from build123d import *

# Parameters (mm, degrees)
SKETCH_1_R          = 1.65
SKETCH_1_R_2        = 4.7
EXTRUDE_1_DEPTH     = 3
FILLET_4_R          = 2
CUT_EXTRUDE_2_DEPTH = 10
SKETCH_3_R          = 1.6
CUT_EXTRUDE_4_DEPTH = 10


with BuildPart() as part:
    # 草图1 → 凸台-拉伸1 (new body)
    with BuildSketch(Plane.XY):
        with BuildLine():
            Line((55.40625, 35), (50.40625, 40))
            Line((50.40625, 40), (0, 40))
            Line((0, 40), (0, 7.5))
            Line((0, 7.5), (30, 0))
            ThreePointArc((30, 0), (37.5, -7.5), (45, 0))
            Line((45, 0), (67.5, 7.5))
            ThreePointArc((67.5, 7.5), (75, 15), (67.5, 22.5))
            Line((67.5, 22.5), (67.5, 35))
            Line((67.5, 35), (55.40625, 35))
        make_face()
        with Locations((8.136085868, 34)):
            Circle(SKETCH_1_R, mode=Mode.SUBTRACT)
        with Locations((42.401142919, 27.875)):
            Circle(SKETCH_1_R, mode=Mode.SUBTRACT)
        with Locations((34.401142919, 27.875)):
            Circle(SKETCH_1_R, mode=Mode.SUBTRACT)
        with Locations((55.40625, 27.875)):
            Circle(SKETCH_1_R, mode=Mode.SUBTRACT)
        with Locations((8.136085868, 15.625)):
            Circle(SKETCH_1_R, mode=Mode.SUBTRACT)
        with Locations((34.401142919, 15.625)):
            Circle(SKETCH_1_R, mode=Mode.SUBTRACT)
        with Locations((42.401142919, 15.625)):
            Circle(SKETCH_1_R, mode=Mode.SUBTRACT)
        with Locations((55.40625, 15.625)):
            Circle(SKETCH_1_R, mode=Mode.SUBTRACT)
        with Locations((8.136085868, 21.75)):
            Circle(SKETCH_1_R, mode=Mode.SUBTRACT)
        with Locations((8.136085868, 27.875)):
            Circle(SKETCH_1_R, mode=Mode.SUBTRACT)
        with Locations((37.5, 0)):
            Circle(SKETCH_1_R_2, mode=Mode.SUBTRACT)
        with Locations((67.5, 15)):
            Circle(SKETCH_1_R_2, mode=Mode.SUBTRACT)
    extrude(amount=EXTRUDE_1_DEPTH)

    # 圆角4
    fillet_4_edges = [part.edges().sort_by_distance(p)[0] for p in [
        (55.40625, 35, 1.5),
        (67.5, 35, 1.5),
        (67.5, 22.5, 1.5),
        (67.5, 7.5, 1.5),
        (45, 0, 1.5),
        (30, 0, 1.5),
        (0, 7.5, 1.5),
        (0, 40, 1.5),
        (50.40625, 40, 1.5),
    ]]
    fillet(fillet_4_edges, radius=FILLET_4_R)

    # 草图2 → 切除-拉伸2 (cut)
    with BuildSketch(Plane.XY):
        with BuildLine():
            Line((49.30341073, 36.65), (27.30341073, 36.65))
            ThreePointArc((27.30341073, 36.65), (25.65341073, 35), (27.30341073, 33.35))
            Line((27.30341073, 33.35), (49.30341073, 33.35))
            ThreePointArc((49.30341073, 33.35), (50.95341073, 35), (49.30341073, 36.65))
        make_face()
    extrude(amount=CUT_EXTRUDE_2_DEPTH, mode=Mode.SUBTRACT)

    # 草图3 → 切除-拉伸4 (cut)
    with BuildSketch(Plane.XY):
        with BuildLine():
            ThreePointArc((36.001142919, 19.875), (35.532513769, 21.00637085), (34.401142919, 21.475))
            Line((34.401142919, 21.475), (34.401142919, 19.875))
            Line((34.401142919, 19.875), (36.001142919, 19.875))
        make_face()
        with BuildLine():
            Line((34.401142919, 19.875), (34.401142919, 21.475))
            ThreePointArc((34.401142919, 21.475), (33.269772069, 18.74362915), (36.001142919, 19.875))
            Line((36.001142919, 19.875), (34.401142919, 19.875))
        make_face()
        with BuildLine():
            ThreePointArc((44.001142919, 19.875), (43.532513769, 21.00637085), (42.401142919, 21.475))
            Line((42.401142919, 21.475), (42.401142919, 19.875))
            Line((42.401142919, 19.875), (40.801142919, 19.875))
            ThreePointArc((40.801142919, 19.875), (42.401142919, 18.275), (44.001142919, 19.875))
        make_face()
        with BuildLine():
            Line((42.401142919, 19.875), (42.401142919, 21.475))
            ThreePointArc((42.401142919, 21.475), (41.269772069, 21.00637085), (40.801142919, 19.875))
            Line((40.801142919, 19.875), (42.401142919, 19.875))
        make_face()
        with Locations((55.40625, 19.875)):
            Circle(SKETCH_3_R)
    extrude(amount=CUT_EXTRUDE_4_DEPTH, mode=Mode.SUBTRACT)


solid = part.part
Verification items for the finished model (mm, model axes). A direction names the side the tool comes from. Give positions to 0.01 mm unless a question says otherwise; leave off trailing zeros. Write each loop counter-clockwise with the first axis right and the second up, starting at its lowest first coordinate (ties: lowest second). Pieces come first, ordered by that corner, then holes.
(1) Access from +Z, -Z, +X, -X, +Y, -Y to the whole of each face (thin tool, end or side, straight path). Record for faces 1 (the face through (38, 33.35, 1)), 2 (the face through (55.459, 35.156, 1.521)).
(2) Cross-section at B-B (y = 3). Enter the section's corners in (x, z), plus the area to 3 significant figures.
(3) Gauge pin test, flat ends, axial feed: pin 1 (1 mm diameter, centred on y = -1.5, z = 1, fed in from -X); pin 2 (2 mm diameter, centred on x = 55.41, y = 15.62, fed in from -Z). Record the tip position at first contact, or that the pin passes through.
(4) Mould release check, pull along Y, two halves, no side actions. Record for faces 3 (the face through (67.93, 23.05, 1.52)), 4 (the face through (37, 22, 0)), 5 (the face through (9.023, 35.391, 1.479)): +Y half, -Y half, draft (parallel to the pull), parting line (faces both ways), or undercut.
(5) Material ranges on line 1 (X direction, y = 21, z = 0.25); line 2 (X direction, y = 17, z = 0.7); line 3 (X direction, y = 31.5, z = 0.3), recorded low to high.
(6) Cross-section at C-C (x = 48.5). Enter the section's corners in (y, z), plus the area to 3 significant figures.
(7) Cross-section at A-A (x = 37.5). Enter the section's corners in (y, z), plus the area to 3 significant figures.
(8) Cross-section at D-D (y = 27). Enter the section's corners in (x, z).
Worked out:
1. face 1: +Z, -Z
1. face 2: +Z, -Z, +X, +Y
2. outline: (18, 0) - (33.88, 0) - (33.88, 3) - (18, 3) - close; (41.12, 0) - (54, 0) - (54, 3) - (41.12, 3) - close
2. area: 86.3 mm2
3. pin 1: stops at x = 30.04
3. pin 2: passes through
4. face 3: +Y half
4. face 4: draft
4. face 5: undercut
5. line 1: x = 0 to 6.67, 9.61 to 33.26, 35.54 to 41.26, 43.54 to 54.27, 56.54 to 72
5. line 2: x = 0 to 7.22, 9.05 to 33.49, 35.31 to 41.49, 43.31 to 54.49, 56.32 to 63.25, 71.75 to 74.73
5. line 3: x = 0 to 67.5
6. outline: (1.17, 0) - (33.35, 0) - (33.35, 3) - (1.17, 3) - close; (36.65, 0) - (40, 0) - (40, 3) - (36.65, 3) - close
6. area: 107 mm2
7. outline: (-7.5, 0) - (-4.7, 0) - (-4.7, 3) - (-7.5, 3) - close; (4.7, 0) - (33.35, 0) - (33.35, 3) - (4.7, 3) - close; (36.65, 0) - (40, 0) - (40, 3) - (36.65, 3) - close
7. area: 104 mm2
8. outline: (0, 0) - (6.74, 0) - (6.74, 3) - (0, 3) - close; (9.53, 0) - (33, 0) - (33, 3) - (9.53, 3) - close; (35.8, 0) - (41, 0) - (41, 3) - (35.8, 3) - close; (43.8, 0) - (54.01, 0) - (54.01, 3) - (43.8, 3) - close; (56.81, 0) - (67.5, 0) - (67.5, 3) - (56.81, 3) - close
